```python
from build123d import *

# Parameters (mm, degrees)
F0_W     = 12
F0_H     = 12
F1_DEPTH = 8


with BuildPart() as f1:
    # F0 (on Top) → F1 (new body)
    with BuildSketch(Plane.XY):
        Polygon((-199.250624, -177.360311), (252.749376, -177.360311), (252.749376, 322.639689), (212.749376, 322.639689), (212.749376, -137.360311), (26.749376, -137.360311), (-159.250624, -137.360311), (-159.250624, 362.639689), (-199.250624, 362.639689), align=None)
        Polygon((-179.250624, -163.360311), (-179.250624, -157.360311), (-185.250624, -157.360311), (-185.250624, -145.360311), (-173.250624, -145.360311), (-173.250624, -151.360311), (-167.250624, -151.360311), (-167.250624, -163.360311), align=None, mode=Mode.SUBTRACT)
        with Locations((-179.250624, -51.360311)):
            Rectangle(F0_W, F0_H, mode=Mode.SUBTRACT)
        with Locations((-73.250624, -157.360311)):
            Rectangle(F0_W, F0_H, mode=Mode.SUBTRACT)
        with Locations((-179.250624, 48.639689)):
            Rectangle(F0_W, F0_H, mode=Mode.SUBTRACT)
        Polygon((20.749376, -151.360311), (26.749376, -151.360311), (32.749376, -151.360311), (32.749376, -163.360311), (20.749376, -163.360311), align=None, mode=Mode.SUBTRACT)
        with Locations((126.749376, -157.360311)):
            Rectangle(F0_W, F0_H, mode=Mode.SUBTRACT)
        with Locations((226.749376, -157.360311)):
            Rectangle(F0_W, F0_H, mode=Mode.SUBTRACT)
        with Locations((-179.250624, 148.639689)):
            Rectangle(F0_W, F0_H, mode=Mode.SUBTRACT)
        with Locations((-179.250624, 248.639689)):
            Rectangle(F0_W, F0_H, mode=Mode.SUBTRACT)
        with Locations((-179.250624, 348.639689)):
            Rectangle(F0_W, F0_H, mode=Mode.SUBTRACT)
    extrude(amount=F1_DEPTH)


solid = f1.part
```
Source: CAD feature listing. Evaluate the final solid. Frame: model axes, mm. Give positions to 0.01 mm unless a question says otherwise; leave off trailing zeros. Loops run counter-clockwise (first coordinate to the right, second up) from the corner with the lowest first, then second, coordinate; pieces in that order, holes last. Notation, with made-up numbers: M -15,-34 L 20,-34 A11 cw 20,-23 Z; hole C -33.5,-24 d10. An arc over 180 degrees is marked long. Put each result on its own line as item: value.
Q1. Section A-A (y = 265). Return the cut outline in (x, z).
Response values:
outline: M -199.25,0 L -159.25,0 L -159.25,8 L -199.25,8 Z; M 212.75,0 L 252.75,0 L 252.75,8 L 212.75,8 Z
Q2. Section C-C (x = 79). Return the cut outline in (y, z), and give its area (3 significant figures).
Response values:
outline: M -177.36,0 L -137.36,0 L -137.36,8 L -177.36,8 Z
area: 320 mm²
Q3. Pin query (flat end, axial travel): P1, Ø4, axis at x = -8, z = 5.5, coming from the +Y side. Return the tip coordinate at first contact, or that it passes through.
Response values:
P1: stops at y = -137.36
Q4. Line query: probe 1 along X at (y, z) = (51, 4); probe 2 along X at (y, z) = (-127, 4.25); probe 3 along Y at (x, z) = (-170, 7.25). Output: solid intervals per line, ascending. Write a range as [from, to].
Response values:
probe 1: x = [-199.25, -185.25], [-173.25, -159.25], [212.75, 252.75]
probe 2: x = [-199.25, -159.25], [212.75, 252.75]
probe 3: y = [-177.36, -163.36], [-151.36, 362.64]
Q5. Section B-B (z = 4.5). Count the separate pieces of the cut face and the enclosed holes in it, and give its area (3 significant figures).
Response values:
separate pieces: 1
enclosed holes: 10
area: 54,900 mm²
